from build123d import *

# Parameters (mm, degrees)
F0_W     = 50
F0_H     = 7
F1_DEPTH = 35
F2_R     = 2.5
F3_DEPTH = 35
F4_R     = 3
F5_R     = 1
F6_DEPTH = 25


with BuildPart() as f1:
    # F0 (on Top) → F1 (new body)
    with BuildSketch(Plane.XY):
        with Locations((0.394545, 0)):
            Rectangle(F0_W, F0_H)
    extrude(amount=F1_DEPTH)

    # F2 (on face) → F3 (cut, through all)
    with BuildSketch(Plane.XY.offset(35)):
        with Locations((-20.605455, 0)):
            Circle(F2_R)
        with Locations((21.394545, 0)):
            Circle(F2_R)
    extrude(amount=-F3_DEPTH, mode=Mode.SUBTRACT)

    # F4
    f4_edges = [f1.edges().sort_by_distance(p)[0] for p in [
        (25.394545, -3.5, 17.5),
        (25.394545, 3.5, 17.5),
        (-24.605455, -3.5, 17.5),
        (-24.605455, 3.5, 17.5),
    ]]
    fillet(f4_edges, radius=F4_R)

    # F5 (on face) → F6 (cut)
    with BuildSketch(Plane.XZ.offset(3.5)):
        with Locations((-4.605455, 20)):
            Circle(F5_R)
    extrude(amount=-F6_DEPTH, mode=Mode.SUBTRACT)


solid = f1.part
Geometry: final body of the model. Coordinates: model frame, mm. Give positions to 0.01 mm unless a question says otherwise; leave off trailing zeros. Loops run counter-clockwise (first coordinate to the right, second up) from the corner with the lowest first, then second, coordinate; pieces in that order, holes last. Notation, with made-up numbers: (-8, 41.5) - (19, 41.5) arc R25 cw to (19, 69.5) - close; hole circle Ø2 at (7.5, 56.5). An arc over 180 degrees is marked (long way). One line per question, with ' | ' between items. Start each with the question number.
(1) Section query B-B on z = 20. Return loops of the section in (x, y).
(2) Section query C-C on x = -4.5. Return loops of the section in (y, z), then the cut area to 3 significant figures.
(3) Section query D-D on y = -3. Return loops of the section in (x, z), then the cut area to 3 significant figures.
(4) Contact query for a flat-ended pin moving along its axis: pin 1 (2.5 mm diameter, centred on x = -4.61, z = 20, fed in from -Y). Output: stop coordinate, or through.
(5) Ray query, line 1 (X direction, y = 2.25, z = 11); line 2 (X direction, y = -1.25, z = 31); line 3 (Y direction, x = 23, z = 23.5). Return the intervals inside material, ascending. Write a range as from..to.
(6) Section query A-A on y = 0. Return loops of the section in (x, z).
(7) Pull-direction query (Z, two-part tool) for faces 1 (the cylindrical face through (-4.144, -0.049, 19.113)), 2 (the flat face through (0, 0, 0)), 3 (the flat face through (0, 0, 35)), 4 (the flat face through (0, 3.5, 17)); classes: released by +Z, released by -Z, zero draft, split by the parting line, or undercut.
The answers:
1) outline: (-24.61, -0.5) arc R3 ccw to (-21.61, -3.5) - (-5.61, -3.5) - (-5.61, 3.5) - (-21.61, 3.5) arc R3 ccw to (-24.61, 0.5) - close; (-3.61, -3.5) - (22.39, -3.5) arc R3 ccw to (25.39, -0.5) - (25.39, 0.5) arc R3 ccw to (22.39, 3.5) - (-3.61, 3.5) - close; hole circle Ø5 at (-20.61, 0); hole circle Ø5 at (21.39, 0)
2) outline: (-3.5, 0) - (3.5, 0) - (3.5, 19.01) - (-3.5, 19.01) - close; (-3.5, 20.99) - (3.5, 20.99) - (3.5, 35) - (-3.5, 35) - close | area: 231 mm2
3) outline: (-23.26, 0) - (24.05, 0) - (24.05, 35) - (-23.26, 35) - close; hole circle Ø2 at (-4.61, 20) | area: 1,650 mm2
4) pin 1: y = -3.5
5) line 1: -24.04..-21.7, -19.52..20.3, 22.48..24.83 | line 2: -24.51..-22.77, -18.44..19.23, 23.56..25.3 | line 3: -3.44..-1.92, 1.92..3.44
6) outline: (-24.61, 0) - (-23.11, 0) - (-23.11, 35) - (-24.61, 35) - close; (-18.11, 0) - (18.89, 0) - (18.89, 35) - (-18.11, 35) - close; (23.89, 0) - (25.39, 0) - (25.39, 35) - (23.89, 35) - close; hole circle Ø2 at (-4.61, 20)
7) face 1: undercut | face 2: released by -Z | face 3: released by +Z | face 4: zero draft
